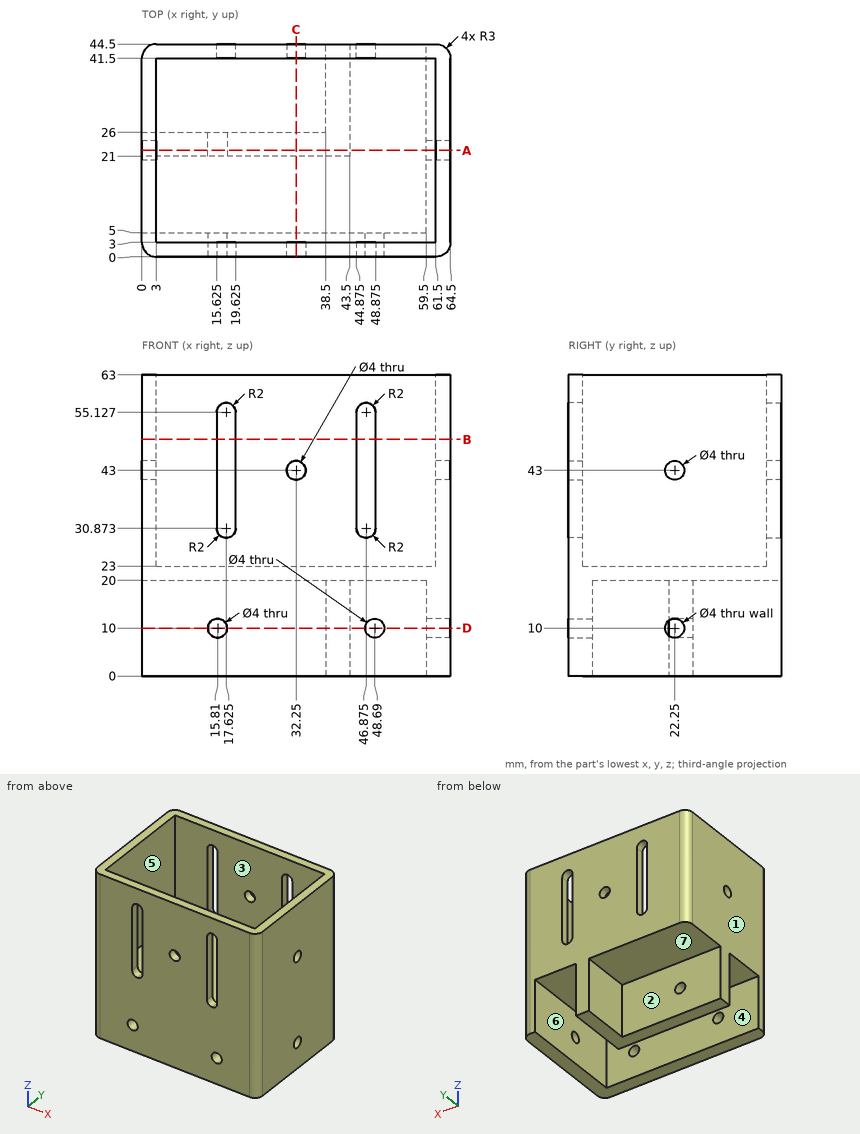
Could you check a few things on this drawing? It's one solid part, dimensions in mm from its lowest x, y, z. A direction names the side the tool comes from. Coordinates: 2 decimals unless noted, no trailing zeros. Write each loop counter-clockwise with the first axis right and the second up, starting at its lowest first coordinate (ties: lowest second). Pieces come first, ordered by that corner, then holes. Notation, with made-up numbers: (12, 6) - (23, 6) arc R34 ccw to (23, 38) - close; hole circle Ø7 at (-37.5, 60). An arc over 180 degrees is marked (long way). Return JSON: item names as keys, results as strings. Group by question number.
Item 1: I'm going to push flat-ended pins straight in: pin 1 Ø5 at (x, y) = (31, 29) entering from +Z; pin 2 Ø16 at (x, z) = (29, 8.5) entering from +Y; pin 3 Ø3 at (x, y) = (25, 36.5) entering from -Z; pin 4 Ø2.5 at (x, z) = (32.25, 43) entering from +Y. Where does each tip first touch, or does it pass through?
Item 2: If we section it at D-D (z = 10): Count the separate pieces of the cut face and the enclosed holes in it, then the cut area to 3 significant figures.
Item 3: If we section it at C-C (x = 32.25): Write out the boundary of the cut face in (y, z).
Item 4: Please list where these lines run through material, in increasing order: probe 1 along Z at (x, y) = (62, 22) (1 decimal); probe 2 along Y at (x, z) = (52, 55.5); probe 3 along X at (y, z) = (4.5, 37).
Item 5: If we section it at A-A (y = 22.25): Write out the boundary of the cut face in (x, z), then the cut area to 3 significant figures.
Item 6: If we section it at B-B (z = 49.5): Write out the boundary of the cut face in (x, y) (1 decimal).
Item 7: Which directions (+Z, -Z, +X, -X, +Y, -Y) give clear straight access to the entire face, cutting with the end or side of a thin tool? Please do the marked faces 4, 5, 6 and 7.
Item 8: We'd pull the mould along X, two halves only. Please class the marked faces 1, 2 and 3: pulls with the +X half, pulls with the -X half, needs draft (parallel to the pull), parting line crosses it, or undercut.
Return value:
{
 "1": {"pin 1": "stops at z = 23", "pin 2": "stops at y = 26", "pin 3": "stops at z = 20", "pin 4": "passes through"},
 "2": {"separate pieces": "6", "enclosed holes": "0", "area": "744 mm^2"},
 "3": {"outline": "(0, 0) - (5, 0) - (5, 20) - (21, 20) - (21, 0) - (26, 0) - (26, 20) - (44.5, 20) - (44.5, 41) - (41.5, 41) - (41.5, 23) - (3, 23) - (3, 41) - (0, 41) - close; (0, 45) - (3, 45) - (3, 63) - (0, 63) - close; (41.5, 45) - (44.5, 45) - (44.5, 63) - (41.5, 63) - close"},
 "4": {"probe 1": "z = 0 to 8, 12 to 41, 45 to 63", "probe 2": "y = 0 to 3, 41.5 to 44.5", "probe 3": "x = 0 to 3, 61.5 to 64.5"},
 "5": {"outline": "(0, 0) - (43.5, 0) - (43.5, 20) - (59.5, 20) - (59.5, 12) - (64.5, 12) - (64.5, 41) - (61.5, 41) - (61.5, 23) - (3, 23) - (3, 41) - (0, 41) - close; (0, 45) - (3, 45) - (3, 63) - (0, 63) - close; (59.5, 0) - (64.5, 0) - (64.5, 8) - (59.5, 8) - close; (61.5, 45) - (64.5, 45) - (64.5, 63) - (61.5, 63) - close; hole circle Ø4 at (15.81, 10)", "area": "1,350 mm^2"},
 "6": {"outline": "(0, 3) arc R3 ccw to (3, 0) - (15.6, 0) - (15.6, 3) - (3, 3) - (3, 41.5) - (15.6, 41.5) - (15.6, 44.5) - (3, 44.5) arc R3 ccw to (0, 41.5) - close; (19.6, 0) - (44.9, 0) - (44.9, 3) - (19.6, 3) - close; (19.6, 41.5) - (44.9, 41.5) - (44.9, 44.5) - (19.6, 44.5) - close; (48.9, 0) - (61.5, 0) arc R3 ccw to (64.5, 3) - (64.5, 41.5) arc R3 ccw to (61.5, 44.5) - (48.9, 44.5) - (48.9, 41.5) - (61.5, 41.5) - (61.5, 3) - (48.9, 3) - close"},
 "7": {"face 4": "-Z, -X", "face 5": "+Z", "face 6": "-Z, +Y", "face 7": "-Z, -X, +Y"},
 "8": {"face 1": "pulls with the -X half", "face 2": "needs draft", "face 3": "undercut"}
}
